Can you work these out from the model? Positions are in its coordinate system, mm. Face numbers are marked on the shaded views. A direction names the side the tool comes from. Round coordinates to 2 decimals unless told otherwise and drop trailing zeros. Order: outer loops, then holes, each group sorted by start corner. A loop starts at its lowest first (then second) coordinate and runs counter-clockwise, first axis right, second up. Notation, with made-up numbers: (73.25, -27) - (109.25, -27) arc R22 cw to (109.25, -4) - close; hole circle Ø3 at (-27, 64.25). An arc over 180 degrees is marked (long way). Write item = value, one per line.
Autodesk Inventor part; units mm, degrees
ref_plane "to_body_XY" through (0, 0, 0) normal (0, -1, 0) x (1, 0, 0)
ref_plane "to_body_YZ" through (0, 0, 0) normal (1, 0, 0) x (0, 0, 1)
ref_plane "to_body_ZX" through (0, 0, 0) normal (0, 0, 1) x (0, -1, 0)
sketch "Sketch_2" plane through (0, 0, 0) normal (1, 0, 0) x (0, 1, 0)
  line L0 (-3.9878, 0) -> (0, 0)
  line L1 (0, 0) -> (0, -5.0038)
  line L2 (0, -5.0038) -> (-3.7338, -5.0038)
  arc A0 (-3.9878, -4.7498) -> (-3.7338, -5.0038) centre (-3.7338, -4.7498) ccw
  line L3 (-3.9878, -4.7498) -> (-3.9878, 0)
  line L4 (-3.9878, 0) -> (0, 0)
revolve "Revolution1" add sketch "Sketch_2" angle 360 about axis through (0, -3.9878, 0) along (0, -1, 0)
sketch "Sketch_4" plane through (0, 0, 0) normal (1, 0, 0) x (0, 1, 0)
  line L0 (-0.254, 0) -> (1.27, 0)
  line L1 (1.27, 0) -> (1.27, -5.7404)
  line L2 (1.27, -5.7404) -> (0.762, -5.7404)
  arc A0 (0.254, -5.2324) -> (0.762, -5.7404) centre (0.762, -5.2324) ccw
  line L3 (0.254, -5.2324) -> (0.254, -4.9784)
  line L4 (0.254, -4.9784) -> (-0.254, -4.9784)
  line L5 (-0.254, -4.9784) -> (-0.254, 0)
  line L6 (-0.254, 0) -> (1.27, 0)
revolve "Revolution2" add sketch "Sketch_4" angle 360 about axis through (0, -0.254, 0) along (0, -1, 0)
ref_plane "to_body_XY" through (0, 0, 0) normal (0, -1, 0) x (1, 0, 0)
ref_plane "to_body_YZ" through (0, 0, 0) normal (1, 0, 0) x (0, 0, 1)
ref_plane "to_body_ZX" through (0, 0, 0) normal (0, 0, 1) x (0, -1, 0)
ref_plane "to_trmnls_XY" through (0, -3.7338, 0) normal (0, 1, 0) x (1, 0, 0)
ref_plane "to_trmnls_YZ" through (0, -3.7338, 0) normal (1, 0, 0) x (0, 0, -1)
ref_plane "to_trmnls_ZX" through (0, -3.7338, 0) normal (0, 0, -1) x (0, 1, 0)
properties part number "SB40-trmnl_hold"
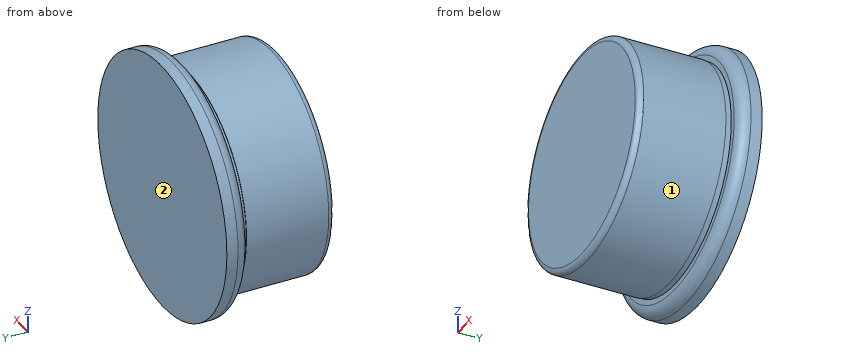
(1) If we section it at D-D (y = 0.6): Write out the boundary of the cut face in (x, z), plus the area to 3 significant figures.
Computed:
outline = circle Ø11.43 at (0, 0)
area = 103 mm^2
(2) If we section it at C-C (y = -1.6): Write out the boundary of the cut face in (x, z), plus the area to 3 significant figures.
Computed:
outline = circle Ø10.01 at (0, 0)
area = 78.7 mm^2
(3) On a 3-axis mill with a long thin cutter (end or side, diameter ignored), from which of +Z, -Z, +X, -X, +Y, -Y can I reach the whole of each face in a straight line? I mean the marked faces 1 and 2. Say none if no direction works.
Computed:
face_1 = -Y
face_2 = +Z, -Z, +X, -X, +Y
(4) If I drill on line 1 (Z direction, x = 0.5, y = -2.85); line 2 (X direction, y = -1, z = 0); line 3 (Z direction, x = -4, y = 0.6), over which ranges is the centre line in solid material (lowest first)? Write a range as from..to.
Computed:
line_1 = -4.98..4.98
line_2 = -5..5
line_3 = -4.08..4.08
(5) Will this pin go through, and if not, where does the flat tip stop? P1, Ø1, axis at y = -2, z = 0.5, coming from the +X side.
Computed:
P1 = 5
